Geometry check sheet. Reference: the model listing, model coordinates, mm. A direction names the side the tool comes from. Round coordinates to 2 decimals unless told otherwise and drop trailing zeros. Loops run counter-clockwise (first coordinate to the right, second up) from the corner with the lowest first, then second, coordinate; pieces in that order, holes last. Notation, with made-up numbers: (-19.75, 27) - (28.25, 27) arc R26 cw to (28.25, 55) - close; hole circle Ø3 at (-12, 84.25). An arc over 180 degrees is marked (long way). Write item = value, one per line.
```python
from build123d import *

# Parameters (mm, degrees)
F1_START = 25
F0_R     = 2.5
F1_DEPTH = 10
F2_R     = 5


with BuildPart() as f1:
    # F0 (on Top) → F1 (new body)
    with BuildSketch(Plane.XY.offset(F1_START)):
        with BuildLine():
            Line((28.115, 28.115), (-28.115, 28.115))
            Line((-28.115, 28.115), (-28.115, 7.6560907126))
            ThreePointArc((-28.115, 7.6560907126), (-22.7514332101, 7.7037324483), (-18.5240804258, 4.4022771811))
            ThreePointArc((-18.5240804258, 4.4022771811), (0, 19.04), (18.5240804258, 4.4022771811))
            ThreePointArc((18.5240804258, 4.4022771811), (22.7514332101, 7.7037324483), (28.115, 7.6560907126))
            Line((28.115, 7.6560907126), (28.115, 28.115))
        make_face()
        with Locations((-23.62, 23.62)):
            Circle(F0_R, mode=Mode.SUBTRACT)
        with Locations((23.62, 23.62)):
            Circle(F0_R, mode=Mode.SUBTRACT)
        with BuildLine():
            Line((-28.115, 2.0247777656), (-28.115, 7.6560907126))
            ThreePointArc((-28.115, 7.6560907126), (-33.5, 0), (-28.115, -7.6560907126))
            Line((-28.115, -7.6560907126), (-28.115, -2.0247777656))
            ThreePointArc((-28.115, -2.0247777656), (-28.78, 0), (-28.115, 2.0247777656))
        make_face()
        with BuildLine():
            ThreePointArc((-18.5240804258, 4.4022771811), (-22.7514332101, 7.7037324483), (-28.115, 7.6560907126))
            Line((-28.115, 7.6560907126), (-28.115, 2.0247777656))
            ThreePointArc((-28.115, 2.0247777656), (-24.2994074418, 3.2444934119), (-21.95, 0))
            ThreePointArc((-21.95, 0), (-24.2994074418, -3.2444934119), (-28.115, -2.0247777656))
            Line((-28.115, -2.0247777656), (-28.115, -7.6560907126))
            ThreePointArc((-28.115, -7.6560907126), (-22.7514332101, -7.7037324483), (-18.5240804258, -4.4022771811))
            ThreePointArc((-18.5240804258, -4.4022771811), (-19.04, 0), (-18.5240804258, 4.4022771811))
        make_face()
        with BuildLine():
            ThreePointArc((-18.5240804258, -4.4022771811), (-22.7514332101, -7.7037324483), (-28.115, -7.6560907126))
            Line((-28.115, -7.6560907126), (-28.115, -28.115))
            Line((-28.115, -28.115), (-7.6560907126, -28.115))
            ThreePointArc((-7.6560907126, -28.115), (-7.7037324483, -22.7514332101), (-4.4022771811, -18.5240804258))
            ThreePointArc((-4.4022771811, -18.5240804258), (-13.4633131138, -13.4633131138), (-18.5240804258, -4.4022771811))
        make_face()
        with Locations((-23.62, -23.62)):
            Circle(F0_R, mode=Mode.SUBTRACT)
        with BuildLine():
            Line((28.115, 2.0247777656), (28.115, 7.6560907126))
            ThreePointArc((28.115, 7.6560907126), (22.7514332101, 7.7037324483), (18.5240804258, 4.4022771811))
            ThreePointArc((18.5240804258, 4.4022771811), (18.9105802569, 2.2162026862), (19.04, 0))
            ThreePointArc((19.04, 0), (18.9105802569, -2.2162026862), (18.5240804258, -4.4022771811))
            ThreePointArc((18.5240804258, -4.4022771811), (22.7514332101, -7.7037324483), (28.115, -7.6560907126))
            Line((28.115, -7.6560907126), (28.115, -2.0247777656))
            ThreePointArc((28.115, -2.0247777656), (21.95, 0), (28.115, 2.0247777656))
        make_face()
        with BuildLine():
            ThreePointArc((33.5, 0), (32.0189264724, 4.6801161845), (28.115, 7.6560907126))
            Line((28.115, 7.6560907126), (28.115, 2.0247777656))
            ThreePointArc((28.115, 2.0247777656), (28.6094934119, 1.0655925582), (28.78, 0))
            ThreePointArc((28.78, 0), (28.6094934119, -1.0655925582), (28.115, -2.0247777656))
            Line((28.115, -2.0247777656), (28.115, -7.6560907126))
            ThreePointArc((28.115, -7.6560907126), (32.0189264724, -4.6801161845), (33.5, 0))
        make_face()
        with BuildLine():
            Line((28.115, -28.115), (28.115, -7.6560907126))
            ThreePointArc((28.115, -7.6560907126), (22.7514332101, -7.7037324483), (18.5240804258, -4.4022771811))
            ThreePointArc((18.5240804258, -4.4022771811), (13.4633131138, -13.4633131138), (4.4022771811, -18.5240804258))
            ThreePointArc((4.4022771811, -18.5240804258), (7.1411046018, -21.4684823155), (8.135, -25.365))
            ThreePointArc((8.135, -25.365), (8.0143784209, -26.7606946394), (7.6560907126, -28.115))
            Line((7.6560907126, -28.115), (28.115, -28.115))
        make_face()
        with Locations((23.62, -23.62)):
            Circle(F0_R, mode=Mode.SUBTRACT)
        with BuildLine():
            ThreePointArc((4.4022771811, -18.5240804258), (0, -19.04), (-4.4022771811, -18.5240804258))
            ThreePointArc((-4.4022771811, -18.5240804258), (-7.7037324483, -22.7514332101), (-7.6560907126, -28.115))
            Line((-7.6560907126, -28.115), (-2.0247777656, -28.115))
            ThreePointArc((-2.0247777656, -28.115), (-1.5407155692, -22.3173089831), (3.415, -25.365))
            ThreePointArc((3.415, -25.365), (3.0476910169, -26.9057155692), (2.0247777656, -28.115))
            Line((2.0247777656, -28.115), (7.6560907126, -28.115))
            ThreePointArc((7.6560907126, -28.115), (8.0143784209, -26.7606946394), (8.135, -25.365))
            ThreePointArc((8.135, -25.365), (7.1411046018, -21.4684823155), (4.4022771811, -18.5240804258))
        make_face()
        with BuildLine():
            Line((-2.0247777656, -28.115), (-7.6560907126, -28.115))
            ThreePointArc((-7.6560907126, -28.115), (0, -33.5), (7.6560907126, -28.115))
            Line((7.6560907126, -28.115), (2.0247777656, -28.115))
            ThreePointArc((2.0247777656, -28.115), (0, -28.78), (-2.0247777656, -28.115))
        make_face()
    extrude(amount=F1_DEPTH)

    # F2
    f2_edges = [f1.edges().sort_by_distance(p)[0] for p in [
        (-28.115, -28.115, 30),
        (28.115, -28.115, 30),
        (28.115, 28.115, 30),
        (-28.115, 28.115, 30),
    ]]
    fillet(f2_edges, radius=F2_R)


solid = f1.part
```
(1) Gauge pin test, flat ends, axial feed: pin 1 (5 mm diameter, centred on y = -16.5, z = 28.5, fed in from -X) (3 decimals); pin 2 (3 mm diameter, centred on y = 13, z = 30.5, fed in from +X) (3 decimals); pin 3 (8 mm diameter, centred on x = 0, y = -25.365, fed in from -Z); pin 4 (1 mm diameter, centred on x = -15, z = 32, fed in from -Y) (3 decimals). Record the tip position at first contact, or that the pin passes through.
Answers follow:
pin_1 = -28.115
pin_2 = 28.115
pin_3 = 25
pin_4 = -28.115
(2) Section check A-A (x = 0). Enter the section's corners in (y, z) (3 decimals), then the cut area to 3 significant figures.
Answers follow:
outline = (-33.5, 25) - (-28.78, 25) - (-28.78, 35) - (-33.5, 35) - close; (-21.95, 25) - (-19.04, 25) - (-19.04, 35) - (-21.95, 35) - close; (19.04, 25) - (28.115, 25) - (28.115, 35) - (19.04, 35) - close
area = 167 mm²
(3) Set-up check for faces 1 (the flat face through (-28.115, 15, 30)), 2 (the flat face through (15, -28.115, 30)), 3 (the flat face through (-28.115, -15, 30)): record each of +Z, -Z, +X, -X, +Y, -Y from which the full face is reachable in a straight line by a thin tool's end or side.
Answers follow:
face_1 = +Z, -Z, -X, +Y
face_2 = +Z, -Z, +X, -Y
face_3 = +Z, -Z, -X, -Y
(4) Section check C-C (x = 25). Enter the section's corners in (y, z).
Answers follow:
outline = (-27.75, 25) - (-25.7, 25) - (-25.7, 35) - (-27.75, 35) - close; (-21.54, 25) - (-3.4, 25) - (-3.4, 35) - (-21.54, 35) - close; (3.4, 25) - (21.54, 25) - (21.54, 35) - (3.4, 35) - close; (25.7, 25) - (27.75, 25) - (27.75, 35) - (25.7, 35) - close
(5) Scan lines: L1, parallel to Y at x = 25.5, z = 28; L2, parallel to Y at x = -0.5, z = 27.25 (3 decimals); L3, parallel to Y at x = 23.62, z = 29.25. Record each from-to range of solid material in increasing order. Write a range as [from, to].
Answers follow:
L1 = [-27.51, -25.27], [-21.97, -3.41], [3.41, 21.97], [25.27, 27.51]
L2 = [-33.485, -28.743], [-21.987, -19.033], [19.033, 28.115]
L3 = [-28.09, -26.12], [-21.12, -2.94], [2.94, 21.12], [26.12, 28.09]
(6) Section check D-D (x = -13). Enter the section's corners in (y, z) (3 decimals).
Answers follow:
outline = (-28.115, 25) - (-13.911, 25) - (-13.911, 35) - (-28.115, 35) - close; (13.911, 25) - (28.115, 25) - (28.115, 35) - (13.911, 35) - close
(7) Mould release check, pull along X, two halves, no side actions. Record for faces 4 (the cylindrical face through (26.005, 24.371, 29.93)), 5 (the cylindrical face through (-26.6, 26.7, 30.1)), 6 (the flat face through (0, 28.115, 30)): pulls with the +X half, pulls with the -X half, needs draft (parallel to the pull), parting line crosses it, or undercut.
Answers follow:
face_4 = undercut
face_5 = pulls with the -X half
face_6 = needs draft
(8) Section check B-B (y = 5.5). Enter the section's corners in (x, z), then the cut area to 3 significant figures.
Answers follow:
outline = (-31.36, 25) - (-18.23, 25) - (-18.23, 35) - (-31.36, 35) - close; (18.23, 25) - (31.36, 25) - (31.36, 35) - (18.23, 35) - close
area = 263 mm²
